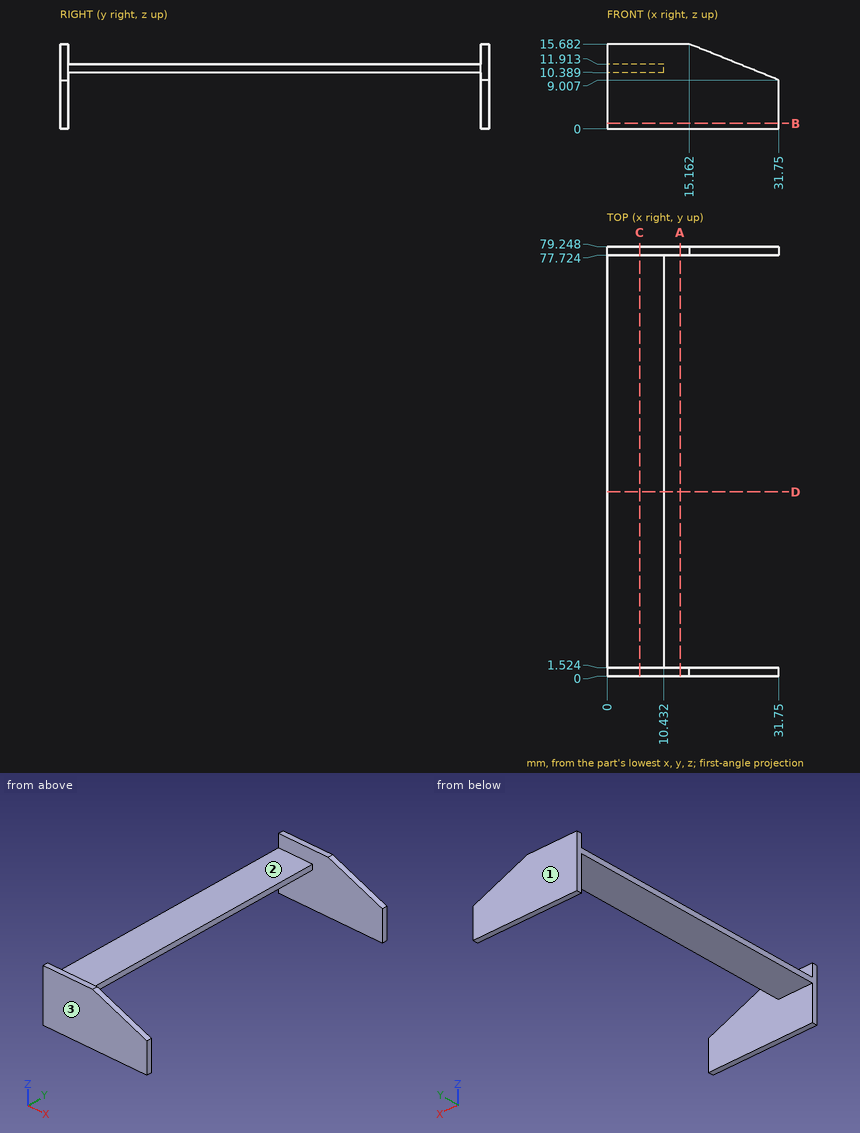
Input: dimensioned drawing with shaded views. Units: mm. Origin: part minimum x, y, z. Give positions to 0.01 mm unless a question says otherwise; leave off trailing zeros. Order: outer loops, then holes, each group sorted by start corner. A loop starts at its lowest first (then second) coordinate and runs counter-clockwise, first axis right, second up.
(1) Section query A-A (x = 13.5). Return the cut outline in (y, z).
(2) Contact query for flat-ended pins moving along their axis: P1, Ø1.5, axis at x = 4.5, y = 27.5, coming from the -Z side; P2, Ø0.8, axis at y = 22.5, z = 11, coming from the +X side; P3, Ø5, axis at x = 3.5, y = 25, coming from the +Z side. Output: stop coordinate, or through.
(3) Material intervals for line 1 along Y through (x, z) = (20.5, 11.5); line 2 along Z through (x, y) = (2, 8); line 3 along X through (y, z) = (37, 11.75), sorted ascending.
(4) Section query D-D (y = 34). Return the cut outline in (x, z), plus the area to 3 significant figures.
(5) Section query C-C (x = 6). Return the cut outline in (y, z).
(6) Pull-direction query (Y, two-part tool) for the marked faces 1, 2 and 3; classes: +Y half, -Y half, draft (parallel to the pull), parting line (faces both ways), or undercut.
(7) Section query B-B (z = 1). Return the cut outline in (x, y).
Outcome:
1. outline: (0, 0) - (1.52, 0) - (1.52, 15.68) - (0, 15.68) - close; (77.72, 0) - (79.25, 0) - (79.25, 15.68) - (77.72, 15.68) - close
2. P1: stops at z = 10.39
2. P2: stops at x = 10.43
2. P3: stops at z = 11.91
3. line 1: y = 0 to 1.52, 77.72 to 79.25
3. line 2: z = 10.39 to 11.91
3. line 3: x = 0 to 10.43
4. outline: (0, 10.39) - (10.43, 10.39) - (10.43, 11.91) - (0, 11.91) - close
4. area: 15.9 mm2
5. outline: (0, 0) - (1.52, 0) - (1.52, 10.39) - (77.72, 10.39) - (77.72, 0) - (79.25, 0) - (79.25, 15.68) - (77.72, 15.68) - (77.72, 11.91) - (1.52, 11.91) - (1.52, 15.68) - (0, 15.68) - close
6. face 1: +Y half
6. face 2: undercut
6. face 3: -Y half
7. outline: (0, 0) - (31.75, 0) - (31.75, 1.52) - (0, 1.52) - close; (0, 77.72) - (31.75, 77.72) - (31.75, 79.25) - (0, 79.25) - close
